from build123d import *

# Parameters (mm, degrees)
BOSS_EXTRUDE1_DEPTH = 1.5875


with BuildPart() as part:
    # Sketch1 → Boss-Extrude1 (new body)
    with BuildSketch(Plane.XY):
        Polygon((6607.534727104, 2635.321979213), (6607.534727104, 2638.496979213), (6555.452027104, 2638.496979213), (6555.452027104, 2635.321979213), (6552.277027104, 2635.321979213), (6552.277027104, 2638.496979213), (6503.374423235, 2638.496979213), (6503.374423235, 2635.321979213), (6500.199423235, 2635.321979213), (6500.199423235, 2638.496979213), (6446.524127104, 2638.496979213), (6446.524127104, 2635.321979213), (6439.716927104, 2635.321979213), (6439.716927104, 2626.127179213), (6614.341927104, 2626.127179213), (6614.341927104, 2635.321979213), align=None)
        Polygon((6531.000725169, 2632.557666317), (6527.825725169, 2634.390753422), (6524.650725169, 2632.557666317), (6524.650725169, 2628.891492108), (6527.825725169, 2627.058405003), (6531.000725169, 2628.891492108), align=None, mode=Mode.SUBTRACT)
        Polygon((6452.874127104, 2632.557666317), (6449.699127104, 2634.390753422), (6446.524127104, 2632.557666317), (6446.524127104, 2628.891492108), (6449.699127104, 2627.058405003), (6452.874127104, 2628.891492108), align=None, mode=Mode.SUBTRACT)
        Polygon((6607.534727104, 2632.557666317), (6604.359727104, 2634.390753422), (6601.184727104, 2632.557666317), (6601.184727104, 2628.891492108), (6604.359727104, 2627.058405003), (6607.534727104, 2628.891492108), align=None, mode=Mode.SUBTRACT)
    extrude(amount=BOSS_EXTRUDE1_DEPTH)


solid = part.part
Can you work these out from the model? Positions are in its coordinate system, mm. Coordinates: 2 decimals unless noted, no trailing zeros. Write each loop counter-clockwise with the first axis right and the second up, starting at its lowest first coordinate (ties: lowest second). Pieces come first, ordered by that corner, then holes. Notation, with made-up numbers: (27.5, 47.5) -> (33.5, 47.5) arc R12 cw to (33.5, 53.5) -> close; hole circle Ø8 at (-26.5, -32). An arc over 180 degrees is marked (long way). Write each question's results on one line, items separated by ' | '. Start each with the question number.
Q1. Imagine slicing it at C-C (x = 6529.5). Write out the boundary of the cut face in (y, z).
Q2. Imagine slicing it at B-B (y = 2630.5). Write out the boundary of the cut face in (x, z), then the cut area to 3 significant figures.
Q3. If I drill on probe 1 along X at (y, z) = (2637.5, 1.55); probe 2 along X at (y, z) = (2632, 0.6); probe 3 along X at (y, z) = (2628.25, 0.8), over which ranges is the centre line in solid material (lowest first)?
Q4. I'm going to push flat-ended pins straight in: pin 1 (0.5 mm diameter, centred on x = 6502, z = 1, fed in from +Y); pin 2 (0.5 mm diameter, centred on y = 2637, z = 1, fed in from -X); pin 3 (0.5 mm diameter, centred on y = 2636.5, z = 0.5, fed in from +X). Where does each tip first touch, or does it pass through?
Q5. Imagine slicing it at A-A (z = 0.4). State how many separate pieces and enclosed holes the cut face has, then the cut area to 3 significant figures.
Taken from the geometry:
1) outline: (2626.13, 0) -> (2628.03, 0) -> (2628.03, 1.59) -> (2626.13, 1.59) -> close; (2633.42, 0) -> (2638.5, 0) -> (2638.5, 1.59) -> (2633.42, 1.59) -> close
2) outline: (6439.72, 0) -> (6446.52, 0) -> (6446.52, 1.59) -> (6439.72, 1.59) -> close; (6452.87, 0) -> (6524.65, 0) -> (6524.65, 1.59) -> (6452.87, 1.59) -> close; (6531, 0) -> (6601.18, 0) -> (6601.18, 1.59) -> (6531, 1.59) -> close; (6607.53, 0) -> (6614.34, 0) -> (6614.34, 1.59) -> (6607.53, 1.59) -> close | area: 247 mm^2
3) probe 1: x = 6446.52 to 6500.2, 6503.37 to 6552.28, 6555.45 to 6607.53 | probe 2: x = 6439.72 to 6446.52, 6452.87 to 6524.65, 6531 to 6601.18, 6607.53 to 6614.34 | probe 3: x = 6439.72 to 6447.64, 6451.76 to 6525.76, 6529.89 to 6602.3, 6606.42 to 6614.34
4) pin 1: stops at y = 2635.32 | pin 2: stops at x = 6446.52 | pin 3: stops at x = 6607.53
5) separate pieces: 1 | enclosed holes: 3 | area: 1,990 mm^2
